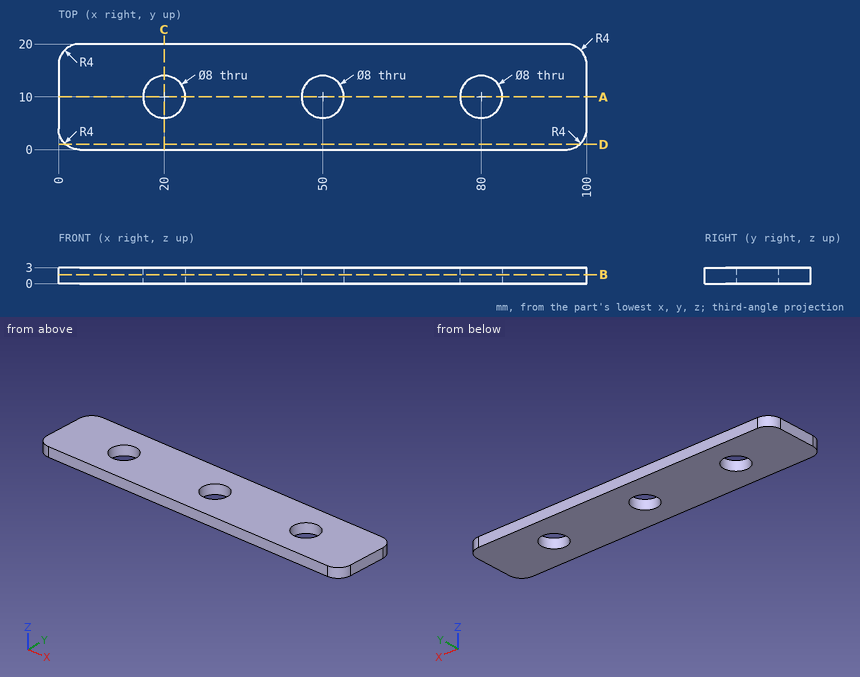
Study the drawing (mm; zero at the part's minimum x, y, z) and answer. Give positions to 0.01 mm unless a question says otherwise; leave off trailing zeros. Order: outer loops, then holes, each group sorted by start corner. A loop starts at its lowest first (then second) coordinate and runs counter-clockwise, first axis right, second up.
1. Section D-D, the plane y = 1 is taken. Determine the outline of the cut face in (x, z), and give its area (3 significant figures).
Result sheet:
outline: (1.35, 0) - (98.65, 0) - (98.65, 3) - (1.35, 3) - close
area: 292 mm2
2. Section B-B, the plane z = 1.7 is taken. Determine the outline of the cut face in (x, y).
Result sheet:
outline: (0, 4) arc R4 ccw to (4, 0) - (96, 0) arc R4 ccw to (100, 4) - (100, 16) arc R4 ccw to (96, 20) - (4, 20) arc R4 ccw to (0, 16) - close; hole circle Ø8 at (20, 10); hole circle Ø8 at (50, 10); hole circle Ø8 at (80, 10)
3. Straight lines are drawn through the part: L1, parallel to X at y = 9.75, z = 0.75; L2, parallel to Y at x = 20, z = 1.1; L3, parallel to X at y = 11, z = 2.5. For each, find the intervals that lie inside material, in ascending order.
Result sheet:
L1: x = 0 to 16.01, 23.99 to 46.01, 53.99 to 76.01, 83.99 to 100
L2: y = 0 to 6, 14 to 20
L3: x = 0 to 16.13, 23.87 to 46.13, 53.87 to 76.13, 83.87 to 100
4. Section C-C, the plane x = 20 is taken. Determine the outline of the cut face in (y, z), and give its area (3 significant figures).
Result sheet:
outline: (0, 0) - (6, 0) - (6, 3) - (0, 3) - close; (14, 0) - (20, 0) - (20, 3) - (14, 3) - close
area: 36.0 mm2
5. Each of these flat-tipped pins is pushed along its axis until it touches: P1, Ø5, axis at x = 24, y = 5.5, coming from the -Z side; P2, Ø1.5, axis at y = 17, z = 1, coming from the +X side. Where does it stop, or does it pass through?
Result sheet:
P1: stops at z = 0
P2: stops at x = 99.99
6. Section A-A, the plane y = 10 is taken. Determine the outline of the cut face in (x, z).
Result sheet:
outline: (0, 0) - (16, 0) - (16, 3) - (0, 3) - close; (24, 0) - (46, 0) - (46, 3) - (24, 3) - close; (54, 0) - (76, 0) - (76, 3) - (54, 3) - close; (84, 0) - (100, 0) - (100, 3) - (84, 3) - close
